Part model, mm, in its own coordinate system. Face numbers are marked on the shaded views. A direction names the side the tool comes from. Coordinates: 2 decimals unless noted, no trailing zeros. Order: outer loops, then holes, each group sorted by start corner. A loop starts at its lowest first (then second) coordinate and runs counter-clockwise, first axis right, second up.
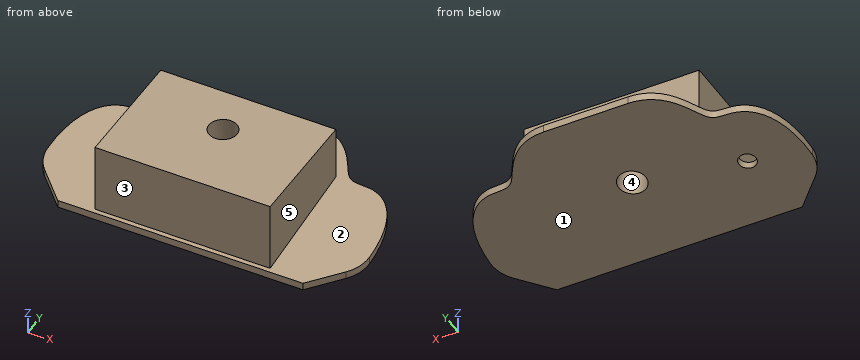
from build123d import *

# Parameters (mm, degrees)
BOSS_EXTRUDE1_START     = -25
BOSS_EXTRUDE1_DEPTH     = 50
CUT_EXTRUDE1_DEPTH      = 341.53226913
CUT_EXTRUDE1_DEPTH_BACK = 341.53226913
BOSS_EXTRUDE2_DEPTH     = 125
CUT_EXTRUDE2_DEPTH      = 356.316937075
CUT_EXTRUDE2_DEPTH_BACK = 356.316937075
SKETCH4_R               = 20
CUT_EXTRUDE3_DEPTH      = 356.316937075
CUT_EXTRUDE3_DEPTH_BACK = 356.316937075
SKETCH6_R               = 12.5


# Read off the part's stored shape, not the designer's step: Boss-Extrude1
with BuildPart() as part:
    # Boss-Extrude1 outline → Boss-Extrude1 (new body)
    with BuildSketch(Plane.XY.offset(BOSS_EXTRUDE1_START)):
        with BuildLine():
            Line((175, 0), (215.218833807, 40.218833807))
            ThreePointArc((215.218833807, 40.218833807), (226.057471223, 56.440000887), (229.863494748, 75.574172084))
            add(Edge.make_bspline(
                [(229.863494748, 75.574172084), (229.863497015, 220.574172084), (130.657195822, 208), (130.657198498, 108), (160, 250), (60, 250)],
                knots=[0, 0, 0, 0, 0, 0, 1, 1, 1, 1, 1, 1], degree=5))
            Line((60, 250), (-60, 250))
            add(Edge.make_bspline(
                [(-60, 250), (-160, 250), (-130.657198498, 108), (-130.657195822, 208), (-229.863497015, 220.574172084), (-229.863494748, 75.574172084)],
                knots=[0, 0, 0, 0, 0, 0, 1, 1, 1, 1, 1, 1], degree=5))
            ThreePointArc((-229.863494748, 75.574172084), (-226.057471223, 56.440000887), (-215.218833807, 40.218833807))
            Line((-215.218833807, 40.218833807), (-175, 0))
            Line((-175, 0), (175, 0))
        make_face()
    extrude(amount=BOSS_EXTRUDE1_DEPTH)

    # Sketch2 → Cut-Extrude1 (cut, two sides: drawn at the far end of the back side and taken through both)
    with BuildSketch(Plane(origin=(0, 0, 0), x_dir=(0, 0, -1), z_dir=(1, 0, 0)).offset(-CUT_EXTRUDE1_DEPTH_BACK)):
        Polygon((23.039732542, -10), (-12.506441807, 260), (35, 260), (35, -10), align=None)
        Polygon((-23.039732542, 260), (12.506441807, -10), (-35, -10), (-35, 260), align=None)
    extrude(amount=CUT_EXTRUDE1_DEPTH + CUT_EXTRUDE1_DEPTH_BACK, mode=Mode.SUBTRACT)

    # Sketch7 → Boss-Extrude2 (add, symmetric)
    with BuildSketch(Plane(origin=(0, 0, 0), x_dir=(0, 0, -1), z_dir=(1, 0, 0))):
        Polygon((-89.599998155, 6), (-89.599998155, 181), (-12.639185232, 181), (10.400001845, 6), align=None)
    extrude(amount=BOSS_EXTRUDE2_DEPTH, both=True)

    # Sketch4 → Cut-Extrude2 (cut, two sides: drawn at the far end of the back side and taken through both)
    with BuildSketch(Plane(origin=(0, 2.811189919, -21.353107392), x_dir=(-1, 0, 0), z_dir=(0, 0.13052619222005532, -0.99144486137381)).offset(-CUT_EXTRUDE2_DEPTH_BACK)):
        with Locations(Location((0, 124.321792579, 0), (0, 0, 90))):
            Circle(SKETCH4_R)
    extrude(amount=CUT_EXTRUDE2_DEPTH + CUT_EXTRUDE2_DEPTH_BACK, mode=Mode.SUBTRACT)

    # Sketch6 → Cut-Extrude3 (cut, two sides: drawn at the far end of the back side and taken through both)
    with BuildSketch(Plane(origin=(0, 2.811189919, -21.353107392), x_dir=(-1, 0, 0), z_dir=(0, 0.13052619222005532, -0.99144486137381)).offset(-CUT_EXTRUDE3_DEPTH_BACK)):
        with Locations(Location((150, 97.164552434, 0), (0, 0, 90))):
            Circle(SKETCH6_R)
    extrude(amount=CUT_EXTRUDE3_DEPTH + CUT_EXTRUDE3_DEPTH_BACK, mode=Mode.SUBTRACT)


solid = part.part
Q1. Cut at B-B on y = 32. Write the cut outline in (x, z).
Results list:
outline: (-207, -17.51) - (207, -17.51) - (207, -6.98) - (125, -6.98) - (125, 89.6) - (-125, 89.6) - (-125, -6.98) - (-207, -6.98) - close
Q2. Cut at A-A on x = -26.5. Write the cut outline in (y, z).
Results list:
outline: (0, -21.72) - (250, 11.19) - (250, 21.72) - (181, 12.64) - (181, 89.6) - (6, 89.6) - (6, -10.4) - (0, -11.19) - close
Q3. Which spindle directions (+Z, -Z, +X, -X, +Y, -Y) get a long thin tool onto all of the face, cutting with end or side? Do the marked faces 1 and 2. Say none if no direction does.
Results list:
face 1: -Z, +X, -X, +Y
face 2: +Z
Q4. Pin check, flat tips, straight feed: pin 1 Ø5 at (x, y) = (11.5, 145) entering from -Z; pin 2 Ø1 at (x, y) = (168, 146.5) entering from -Z; pin 3 Ø8 at (y, z) = (134.5, 77.5) entering from +X. Stop position of each tip, or through.
Results list:
pin 1: stops at z = -2.96
pin 2: stops at z = -2.5
pin 3: stops at x = 125
Q5. Wall check: line 1 along X through (y, z) = (121, 36); line 2 along Y through (x, z) = (23, 66.5); line 3 along X through (y, z) = (26, 9). Give the ranges that are in metal, low to high.
Results list:
line 1: x = -125 to -20, 20 to 125
line 2: y = 6 to 181
line 3: x = -125 to 125
Q6. Mould opens along X. For the marked faces 3, 4 and 5 say: pulls with the +X half, pulls with the -X half, needs draft (parallel to the pull), parting line crosses it, or undercut.
Results list:
face 3: needs draft
face 4: undercut
face 5: pulls with the +X half
